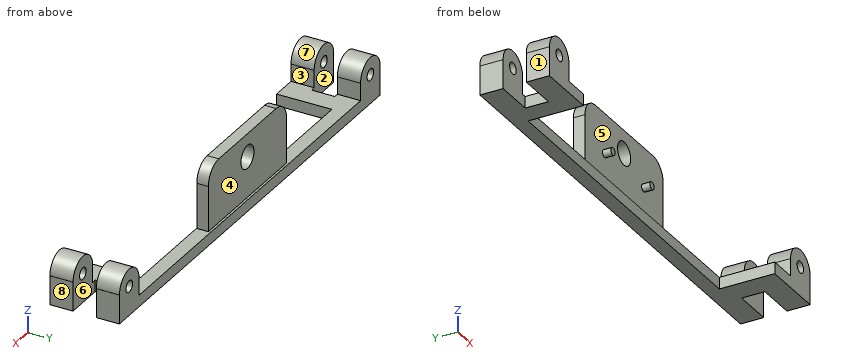
```python
from build123d import *

# Parameters (mm, degrees)
F2_R      = 1.5875
F4_DEPTH  = 9.525
F3_W      = 11.9612812996
F3_H      = 17.3548664898
F5_DEPTH  = 3.175
F6_W      = 38.1
F6_H      = 19.05
F7_DEPTH  = 3.175
F8_R      = 1.016
F9_DEPTH  = 5.471363198
F10_R     = 5.08
F11_W     = 93.1863598526
F11_H     = 18.8650693744
F12_DEPTH = 3.175
F13_R     = 3.175
F14_DEPTH = 9.5102116466


with BuildPart() as f4:
    # F2 (on Front) → F4 (new body, symmetric)
    with BuildSketch(Plane.XZ):
        with BuildLine():
            ThreePointArc((63.4873, 6.3627), (58.7248, 11.1252), (53.9623, 6.3627))
            ThreePointArc((53.9623, 6.3627), (58.7248, 1.6002), (63.4873, 6.3627))
        make_face()
        with Locations((58.7248, 6.3627)):
            Circle(F2_R, mode=Mode.SUBTRACT)
        with BuildLine():
            Line((53.9623, 1.5875), (63.5, 1.5875))
            Line((63.5, 1.5875), (63.5, 6.3627))
            Line((63.5, 6.3627), (63.4873, 6.3627))
            ThreePointArc((63.4873, 6.3627), (58.7248, 1.6002), (53.9623, 6.3627))
            Line((53.9623, 6.3627), (53.9623, 1.5875))
        make_face()
        Polygon((-63.5, 1.5875), (-63.5, -1.5875), (63.5, -1.5875), (63.5, 1.5875), (53.9623, 1.5875), (-53.9623, 1.5875), align=None)
        with BuildLine():
            ThreePointArc((-63.4873, 6.3627), (-58.7248, 1.6002), (-53.9623, 6.3627))
            ThreePointArc((-53.9623, 6.3627), (-58.7248, 11.1252), (-63.4873, 6.3627))
        make_face()
        with Locations((-58.7248, 6.3627)):
            Circle(F2_R, mode=Mode.SUBTRACT)
        with BuildLine():
            Line((-63.5, 6.3627), (-63.5, 1.5875))
            Line((-63.5, 1.5875), (-53.9623, 1.5875))
            Line((-53.9623, 1.5875), (-53.9623, 6.3627))
            ThreePointArc((-53.9623, 6.3627), (-58.7248, 1.6002), (-63.4873, 6.3627))
            Line((-63.4873, 6.3627), (-63.5, 6.3627))
        make_face()
    extrude(amount=F4_DEPTH, both=True)

    # F3 (on Front) → F5 (cut, symmetric)
    with BuildSketch(Plane.XZ):
        with Locations((-58.6804002523, 4.3448181823)):
            Rectangle(F3_W, F3_H)
        with Locations((58.6804002523, 4.3448181823)):
            Rectangle(F3_W, F3_H)
    extrude(amount=F5_DEPTH, both=True, mode=Mode.SUBTRACT)

    # F6 (on offset) → F7 (join)
    with BuildSketch(Plane.XZ.offset(-8.89)):
        with Locations((0, 9.525)):
            Rectangle(F6_W, F6_H)
    extrude(amount=F7_DEPTH)

    # F8 (on offset) → F9 (join)
    with BuildSketch(Plane.XZ.offset(-8.89)):
        with Locations((-9.525, 7.9375)):
            Circle(F8_R)
        with Locations((9.525, 7.9375)):
            Circle(F8_R)
    extrude(amount=F9_DEPTH)

    # F10
    f10_edges = [f4.edges().sort_by_distance(p)[0] for p in [
        (19.05, 7.3025, 19.05),
        (-19.05, 7.3025, 19.05),
    ]]
    fillet(f10_edges, radius=F10_R)

    # F11 (on Top) → F12 (cut, symmetric)
    with BuildSketch(Plane.XY):
        with Locations((-0.332666561, -3.7929313257)):
            Rectangle(F11_W, F11_H)
    extrude(amount=F12_DEPTH, both=True, mode=Mode.SUBTRACT)

    # F13 (on offset) → F14 (cut)
    with BuildSketch(Plane.XZ.offset(-8.89)):
        with Locations((0, 12.7)):
            Circle(F13_R)
    extrude(amount=F14_DEPTH, mode=Mode.SUBTRACT)


solid = f4.part
```
Read the model definition and answer for the solid it produces. Units are mm, in the model's axes. Face numbers are marked on the shaded views. A direction names the side the tool comes from. Give positions to 0.01 mm unless a question says otherwise; leave off trailing zeros. Write each loop counter-clockwise with the first axis right and the second up, starting at its lowest first coordinate (ties: lowest second). Pieces come first, ordered by that corner, then holes. Notation, with made-up numbers: (15, -10) - (46, -10) arc R25 cw to (46, 28) - close; hole circle Ø4 at (-39, 86.5). An arc over 180 degrees is marked (long way). Write item = value, one per line. Start each with the question number.
Item 1: Find section A-A (y = -8). State how many separate pieces and enclosed holes the cut face has, then the cut area to 3 significant figures.
Item 2: Find section B-B (z = 12.7). Give the vertices of the cut face in (x, y) (3 decimals).
Item 3: Find the intervals of material crossed by probe 1 along X at (y, z) = (-7.5, 6.5); probe 2 along X at (y, z) = (3.25, 2.75); probe 3 along X at (y, z) = (-3, 1), in increasing order. Write a range as [from, to].
Item 4: The mould has two halves that part along X. Classify the marked faces 5, 6, 7 and 8: +X half, -X half, draft (parallel to the pull), parting line (faces both ways), or undercut.
Item 5: A tool of negligible diameter and unlimited length cuts with its end or side. For the marked faces 1, 2, 3 and 4, from which of +Z, -Z, +X, -X, +Y, -Y can it reach the whole face along a straight path? Write none if from no direction.
Item 6: Each of these flat-tipped pins is pushed along its axis until it touches: P1, Ø5, axis at x = -4, z = 6.5, coming from the +Y side; P2, Ø1.6, axis at y = 1, z = -0.5, coming from the +X side; P3, Ø1.6, axis at y = -1.5, z = 0, coming from the -X side; P4, Ø8, axis at x = 13.5, y = 5.5, coming from the -Z side. Where does it stop, or does it pass through?
Response:
q1.separate_pieces = 2
q1.enclosed_holes = 2
q1.area = 254 mm²
q2.outline = (-19.05, 5.715) - (-3.175, 5.715) - (-3.175, 8.89) - (-19.05, 8.89) - close; (3.175, 5.715) - (19.05, 5.715) - (19.05, 8.89) - (3.175, 8.89) - close
q3.probe_1 = [-63.49, -60.31], [-57.14, -53.96], [53.96, 57.14], [60.31, 63.49]
q3.probe_2 = [-63.5, -53.96], [53.96, 63.5]
q3.probe_3 = [-52.7, -46.93], [46.26, 52.7]
q4.face_5 = undercut
q4.face_6 = draft
q4.face_7 = undercut
q4.face_8 = +X half
q5.face_1 = +Z, -Z, -X, +Y, -Y
q5.face_2 = +Z, -Z, -X
q5.face_3 = +Z, +Y, -Y
q5.face_4 = +Z, +Y
q6.P1 = 8.89
q6.P2 = 52.7
q6.P3 = -52.7
q6.P4 = -1.59
